Work out the finished part from the listing and answer in its coordinate system (mm). Coordinates: 2 decimals unless noted, no trailing zeros. Order: outer loops, then holes, each group sorted by start corner. A loop starts at its lowest first (then second) coordinate and runs counter-clockwise, first axis right, second up. Notation, with made-up numbers: M 31,25 L 41,25 A6 ccw 41,36 Z; hole C -27,16 d6. An arc over 180 degrees is marked long. Answer in a Markdown table with one row per item. Add a question column.
Item 1: The part is cut by section D-D (z = 6.75). Write down the section's boundary in (x, y), then the cut area to 4 significant figures.
Item 2: Consider line 1 (X direction, y = 0.65, z = 6.75); line 2 (X direction, y = 0.75, z = 35) (3 decimals); line 3 (Z direction, x = 52, y = 1.2). Determine where each line is inside the solid, lowest interval first. Write a range as from..to.
Item 3: The part is cut by section A-A (z = 28). Write down the section's boundary in (x, y) (3 decimals), then the cut area to 3 significant figures.
Item 4: Flat-ended cylindrical pins translate along their axes: pin 1 Ø3.5 at (x, z) = (51.75, 6.75) entering from +Y; pin 2 Ø1.8 at (x, z) = (6.75, 6.75) entering from +Y; pin 3 Ø0.6 at (x, y) = (29, 1.5) entering from +Z. Find the tip coordinate at first contact, or state that the pin passes through.
Item 5: The part is cut by section B-B (x = 51.75). Write down the section's boundary in (y, z), then the cut area to 4 significant figures.
Item 6: The part is cut by section C-C (y = 1.2). Write down the section's boundary in (x, z) (3 decimals).
from build123d import *

# Parameters (mm, degrees)
EXTRUDE_1_DEPTH     = 1.9
CUT_EXTRUDE_1_REACH = 72.058
SKETCH_2_R          = 1.5


with BuildPart() as part:
    # 草图1 → 凸台-拉伸1 (new body)
    with BuildSketch(Plane(origin=(0, 0, 0), x_dir=(1, 0, 0), z_dir=(0, 1, 0))):
        Polygon((0, 0), (58.5, 0), (58.5, -38.5), (39.025, -38.5), (39.025, -18.8), (19.475, -18.8), (19.475, -38.5), (0, -38.5), align=None)
    extrude(amount=EXTRUDE_1_DEPTH)

    # 草图2 → 切除-拉伸1 (cut, up to next)
    with BuildSketch(Plane.XZ, mode=Mode.PRIVATE) as cut_extrude_1_sk1:
        with Locations(Location((51.75, 6.75, 0), (0, 0, 270))):
            Circle(SKETCH_2_R)
    cut_extrude_1_tool1 = extrude(cut_extrude_1_sk1.sketch, amount=-CUT_EXTRUDE_1_REACH, mode=Mode.PRIVATE) & part.part
    # 草图2 → 切除-拉伸1 (cut, up to next)
    with BuildSketch(Plane.XZ, mode=Mode.PRIVATE) as cut_extrude_1_sk2:
        with Locations(Location((6.75, 6.75, 0), (0, 0, 270))):
            Circle(SKETCH_2_R)
    cut_extrude_1_tool2 = extrude(cut_extrude_1_sk2.sketch, amount=-CUT_EXTRUDE_1_REACH, mode=Mode.PRIVATE) & part.part
    add(cut_extrude_1_tool1.solids().sort_by_distance((51.75, 0, 6.75))[0], mode=Mode.SUBTRACT)
    add(cut_extrude_1_tool2.solids().sort_by_distance((6.75, 0, 6.75))[0], mode=Mode.SUBTRACT)


solid = part.part
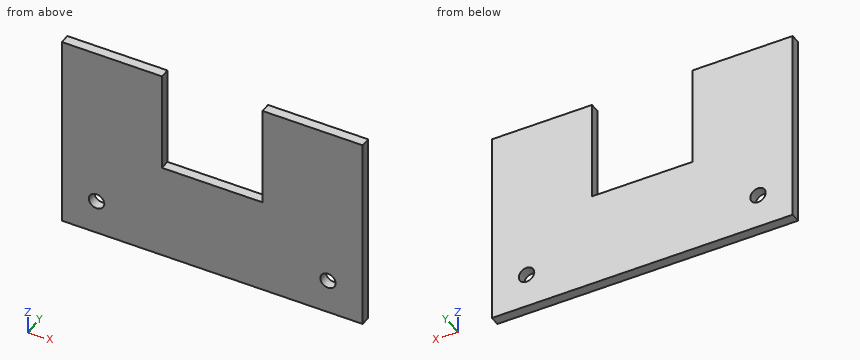
Reply:
| question | item | result |
|---|---|---|
| 1 | outline | M 0,0 L 5.25,0 L 5.25,1.9 L 0,1.9 Z; M 8.25,0 L 50.25,0 L 50.25,1.9 L 8.25,1.9 Z; M 53.25,0 L 58.5,0 L 58.5,1.9 L 53.25,1.9 Z |
| 1 | area | 99.75 mm2 |
| 2 | line 1 | x = 0..5.25, 8.25..50.25, 53.25..58.5 |
| 2 | line 2 | x = 0..19.475, 39.025..58.5 |
| 2 | line 3 | z = 0..5.27, 8.23..38.5 |
| 3 | outline | M 0,0 L 19.475,0 L 19.475,1.9 L 0,1.9 Z; M 39.025,0 L 58.5,0 L 58.5,1.9 L 39.025,1.9 Z |
| 3 | area | 74.0 mm2 |
| 4 | pin 1 | stops at y = 1.9 |
| 4 | pin 2 | passes through |
| 4 | pin 3 | stops at z = 18.8 |
| 5 | outline | M 0,0 L 1.9,0 L 1.9,5.25 L 0,5.25 Z; M 0,8.25 L 1.9,8.25 L 1.9,38.5 L 0,38.5 Z |
| 5 | area | 67.45 mm2 |
| 6 | outline | M 0,0 L 58.5,0 L 58.5,38.5 L 39.025,38.5 L 39.025,18.8 L 19.475,18.8 L 19.475,38.5 L 0,38.5 Z; hole C 6.75,6.75 d3; hole C 51.75,6.75 d3 |
